from build123d import *

# Parameters (mm, degrees)
BOSS_EXTRUDE1_DEPTH = 13
FILLET1_R           = 1
FILLET2_R           = 6
BOSS_EXTRUDE2_START = 7
BOSS_EXTRUDE2_DEPTH = 7
SKETCH3_W           = 17.1
SKETCH3_H           = 5
BOSS_EXTRUDE3_DEPTH = 17.1
FILLET3_R           = 6
SKETCH4_W           = 17.1
SKETCH4_H           = 17.1
BOSS_EXTRUDE4_DEPTH = 20
FILLET4_R           = 2
FILLET6_R           = 1
FILLET7_R           = 1
SKETCH6_R           = 1.9999999999999987
CUT_EXTRUDE1_DEPTH  = 14.000000000000002
FILLET8_R           = 3


with BuildPart() as part:
    # Sketch1 → Boss-Extrude1 (new body)
    with BuildSketch(Plane.XY):
        with BuildLine():
            Line((-0.9999999999999998, 7.433034373659251), (-1.0000000000000002, 12.433034373659252))
            Line((-1.0000000000000002, 12.433034373659252), (-5, 12.433034373659252))
            Line((-5, 12.433034373659252), (-4.999999999999999, 5.590169943749475))
            ThreePointArc((-4.999999999999999, 5.590169943749475), (-1.38e-15, -7.5), (4.999999999999999, 5.5901699437494745))
            Line((4.999999999999999, 5.5901699437494745), (5, 12.433034373659252))
            Line((5, 12.433034373659252), (0.9999999999999998, 12.433034373659252))
            Line((0.9999999999999998, 12.433034373659252), (0.9999999999999993, 7.433034373659251))
            Line((0.9999999999999993, 7.433034373659251), (0.9999999999999998, 2.8284271247461907))
            ThreePointArc((0.9999999999999998, 2.8284271247461907), (-5.5e-16, -3.0000000000000004), (-1.0000000000000002, 2.8284271247461903))
            Line((-1.0000000000000002, 2.8284271247461903), (-0.9999999999999998, 7.433034373659251))
        make_face()
    extrude(amount=BOSS_EXTRUDE1_DEPTH)

    # Fillet1
    fillet1_edges = [part.edges().sort_by_distance(p)[0] for p in [
        (-1.0000000000000004, 2.8284271247461907, 6.5),
        (0.9999999999999998, 2.8284271247461907, 6.5),
        (-4.7e-16, -3.0000000000000004, 13),
    ]]
    fillet(fillet1_edges, radius=FILLET1_R)

    # Fillet2
    fillet2_edges = [part.edges().sort_by_distance(p)[0] for p in [
        (-3, 12.433034373659252, 13),
        (3, 12.433034373659252, 0),
        (-3, 12.433034373659252, 0),
        (3, 12.433034373659252, 13),
    ]]
    fillet(fillet2_edges, radius=FILLET2_R)

    # Sketch2 → Boss-Extrude2 (add)
    with BuildSketch(Plane(origin=(0, 0, 0), x_dir=(-1, 0, 0), z_dir=(0, 0, -1)).offset(BOSS_EXTRUDE2_START)):
        with BuildLine():
            Line((-7.5, 0), (-3.0000000000000004, 0))
            ThreePointArc((-3.0000000000000004, 0), (-5.5e-16, -3.0000000000000004), (3.0000000000000004, 0))
            Line((3.0000000000000004, 0), (7.5, 0))
            ThreePointArc((7.5, 0), (-1.38e-15, -7.5), (-7.5, 0))
        make_face()
    extrude(amount=-BOSS_EXTRUDE2_DEPTH)

    # Sketch3 → Boss-Extrude3 (add)
    with BuildSketch(Plane.XY.offset(13)):
        with Locations((1.78e-15, -7.5)):
            Rectangle(SKETCH3_W, SKETCH3_H)
    extrude(amount=-BOSS_EXTRUDE3_DEPTH)

    # Fillet3
    # the kernel refuses this fillet: 6 mm, written as the material it adds along each edge
    with BuildSketch(Plane(origin=(5.590169943749475, -5, 13), x_dir=(0.407962135259343, 0.9129988478605203, 0), z_dir=(0, 0, -1))) as fillet3_piece_1:
        with BuildLine():
            CenterArc((6.396366403246306, 5.714903515427595), FILLET3_R, 210.13883458163096, 42.12773397862901)
            Line((1.2074985897527464, 2.70232143121967), (1.1037212334828754, 2.642069789535512))
            ThreePointArc((1.1037212334828754, 2.642069789535512), (0.4941894331331104, 1.4001161718409558), (-0.10955986174326253, 0.0489554562311212))
            Line((-0.10955986174326253, 0.0489554562311212), (0.03655066516140769, -0.11429807030855153))
            ThreePointArc((0.03655066516140769, -0.11429807030855153), (2.2844165725879635, 0.23637060571550603), (4.5322824800145245, -0.11429807030855171))
            Line((4.5322824800145245, -0.11429807030855171), (4.568833145175932, -9e-17))
        make_face()
    extrude(amount=17.1)
    with BuildSketch(Plane(origin=(-5.590169943749474, -5, 13), x_dir=(-0.40796213525934283, 0.9129988478605204, 0), z_dir=(0, 0, -1))) as fillet3_piece_2:
        with BuildLine():
            CenterArc((6.396366403246302, -5.714903515427596), FILLET3_R, 107.73343143974, 42.12773397862901)
            Line((1.2074985897527435, -2.702321431219668), (1.1037212334828725, -2.642069789535509))
            ThreePointArc((1.1037212334828725, -2.642069789535509), (0.4941894331331094, -1.4001161718409545), (-0.10955986174326254, -0.04895545623112119))
            Line((-0.10955986174326254, -0.04895545623112119), (0.03655066516140771, 0.11429807030855152))
            ThreePointArc((0.03655066516140771, 0.11429807030855152), (2.284416572587965, -0.23637060571550497), (4.532282480014523, 0.11429807030855221))
            Line((4.532282480014523, 0.11429807030855221), (4.56883314517593, 0))
        make_face()
    extrude(amount=17.1)

    # Sketch4 → Boss-Extrude4 (add)
    with BuildSketch(Plane.XZ.offset(10)):
        with Locations((1.78e-15, 4.45)):
            Rectangle(SKETCH4_W, SKETCH4_H)
    extrude(amount=BOSS_EXTRUDE4_DEPTH)

    # Fillet4
    fillet4_edges = [part.edges().sort_by_distance(p)[0] for p in [
        (8.549999999999962, -17.499999999999645, 13),
        (8.549999999999962, -17.499999999999645, -4.100000000000001),
        (-8.54999999999996, -17.499999999999645, 13),
        (-8.54999999999996, -17.499999999999645, -4.100000000000001),
    ]]
    fillet(fillet4_edges, radius=FILLET4_R)

    # Sketch5 → Revolve1 (revolve)
    with BuildSketch(Plane(origin=(0, 0, 0), x_dir=(0, 0, -1), z_dir=(1, 0, 0))):
        Polygon((6.999999999999999, -8.7e-16), (7.000000000000001, -15), (9.499999999999998, -12.5), (12, -15), (12, 0), align=None)
    revolve(axis=Axis((0, 0, 0), (0, -1.2e-16, -1)))

    # Fillet6
    fillet6_edges = [part.edges().sort_by_distance(p)[0] for p in [
        (4.1e-16, -3, -7),
        (5.25, 0, -7),
        (-1.01e-15, -7.499999999999999, -7),
        (-5.25, 0, -7),
    ]]
    fillet(fillet6_edges, radius=FILLET6_R)

    # Fillet7
    fillet7_edges = [part.edges().sort_by_distance(p)[0] for p in [
        (-1.53e-15, 12.499999999999996, -9.500000000000002),
    ]]
    fillet(fillet7_edges, radius=FILLET7_R)

    # Sketch6 → Cut-Extrude1 (cut)
    with BuildSketch(Plane.ZY.offset(4.999999999999998)):
        with Locations(Location((6.500000000000002, 8.942387299959254, 0), (0, 0, 270))):
            Circle(SKETCH6_R)
    extrude(amount=-CUT_EXTRUDE1_DEPTH, mode=Mode.SUBTRACT)

    # Fillet8
    fillet8_edges = [part.edges().sort_by_distance(p)[0] for p in [
        (5.25, 0, 0),
        (-5.25, 0, 0),
    ]]
    fillet(fillet8_edges, radius=FILLET8_R)


solid = part.part
Could you check a few things on this model? Use its own coordinates, in mm. A direction names the side the tool comes from. Coordinates: 2 decimals unless noted, no trailing zeros. Write each loop counter-clockwise with the first axis right and the second up, starting at its lowest first coordinate (ties: lowest second). Pieces come first, ordered by that corner, then holes. Notation, with made-up numbers: (53.5, -36.75) - (63.5, -36.75) arc R27 ccw to (63.5, 1.25) - close; hole circle Ø3 at (65.5, 36). An arc over 180 degrees is marked (long way). Put each result on its own line as item: value. Start each with the question number.
Q1. Thinking about a two-plate mould opening in Z: for faces 1 (the cylindrical face through (0, -3, 3)), 2 (the cylindrical face through (7.98, -16.68, 12.4)), 3 (the flat face through (-5, 0, -5)), which applies, pulls with the +Z half, pulls with the -Z half, needs draft (parallel to the pull), parting line crosses it, or undercut?
Q2. I want a section at A-A on y = -20. Write out the boundary of the cut face in (x, z).
Q3. I want a section at D-D on y = 7.5. Count the separate pieces of the cut face and the enclosed holes in it, plus the area to 3 significant figures.
Q4. Please list where these lines run through material, in increasing order: L1, parallel to Z at x = 0.5, y = -11; L2, parallel to Z at x = -1, y = -13.5; L3, parallel to Z at x = -3, y = -22.
Q5. Which directions (+Z, -Z, +X, -X, +Y, -Y) give clear straight access to the entire face, cutting with the end or side of a thin tool? Please do faces 4 (the cylindrical face through (-5.133, 0.301, -6.715)), 5 (the conical face through (13, 2.89, -10.32)), 6 (the flat face through (5, 6.7, 6.4)).
Q6. I want a section at C-C on z = 1.75. Write out the boundary of the cut face in (x, y).
Q7. I'm going to push flat-ended pins straight in: P1, Ø1, axis at x = 1, y = -3, coming from the +Z side; P2, Ø2, axis at y = 8.5, z = 6.5, coming from the -X side; P3, Ø0.5, axis at x = 3, z = 6.5, coming from the +Y side; P4, Ø2.5, axis at x = 4, z = -4.5, coming from the +Y side. Where does each tip first touch, or does it pass through?
Q8. I want a section at B-B on z = 6.5. Write out the boundary of the cut face in (x, y), plus the area to 3 significant figures.
Checks:
1. face 1: needs draft
1. face 2: pulls with the +Z half
1. face 3: undercut
2. outline: (-8.55, -2.1) arc R2 ccw to (-6.55, -4.1) - (6.55, -4.1) arc R2 ccw to (8.55, -2.1) - (8.55, 11) arc R2 ccw to (6.55, 13) - (-6.55, 13) arc R2 ccw to (-8.55, 11) - close
3. separate pieces: 5
3. enclosed holes: 0
3. area: 196 mm²
4. L1: -12 to -7, -4.1 to 13
4. L2: -12 to -10.54, -8.46 to -7, -4.1 to 13
4. L3: -4.1 to 13
5. face 4: +X, -X, +Y
5. face 5: none
5. face 6: +Z, +X, +Y
6. outline: (-8.55, -30) - (8.55, -30) - (8.55, -5) arc R6 cw to (7.45, -0.83) arc R7.5 ccw to (5, 5.59) - (5, 10.67) - (1, 10.67) - (1, 3.46) arc R1 ccw to (1.5, 2.6) arc R3 cw (long way) to (-1.5, 2.6) arc R1 ccw to (-1, 3.46) - (-1, 10.67) - (-5, 10.67) - (-5, 5.59) arc R7.5 ccw to (-7.45, -0.83) arc R6 cw to (-8.55, -5) - close
7. P1: z = 12.94
7. P2: through
7. P3: y = 12.43
7. P4: y = 0
8. outline: (-8.55, -30) - (8.55, -30) - (8.55, -5) arc R6 cw to (7.45, -0.83) arc R7.5 ccw to (5, 5.59) - (5, 6.94) - (1, 6.94) - (1, 3.46) arc R1 ccw to (1.5, 2.6) arc R3 cw (long way) to (-1.5, 2.6) arc R1 ccw to (-1, 3.46) - (-1, 6.94) - (-5, 6.94) - (-5, 5.59) arc R7.5 ccw to (-7.45, -0.83) arc R6 cw to (-8.55, -5) - close; (-5, 10.94) - (-1, 10.94) - (-1, 12.43) - (-5, 12.43) - close; (1, 10.94) - (5, 10.94) - (5, 12.43) - (1, 12.43) - close
8. area: 569 mm²
